Part model, mm, in its own coordinate system. Face numbers are marked on the shaded views. Round coordinates to 2 decimals unless told otherwise and drop trailing zeros. Order: outer loops, then holes, each group sorted by start corner. A loop starts at its lowest first (then second) coordinate and runs counter-clockwise, first axis right, second up. Notation, with made-up numbers: M 69.5,30.5 L 90.5,30.5 A34 ccw 90.5,67.5 Z; hole C 64,63 d2. An arc over 180 degrees is marked long. One line per question, with ' | ' between items.
from build123d import *

# Parameters (mm, degrees)
SKETCH_R  = 11
PAD_DEPTH = 7
FILLET_R  = 2


with BuildPart() as part:
    # Sketch → Pad (new body)
    with BuildSketch(Plane.XY):
        with BuildLine():
            ThreePointArc((-7.384634, -14.193914), (0, -16), (7.384634, -14.193914))
            ThreePointArc((16.615361, -14.193911), (11.999997, -13.065125), (7.384634, -14.193914))
            ThreePointArc((16.615361, -14.193911), (40, 0), (16.615361, 14.193911))
            ThreePointArc((7.384634, 14.193914), (11.999997, 13.065125), (16.615361, 14.193911))
            ThreePointArc((7.384634, 14.193914), (0, 16), (-7.384634, 14.193914))
            ThreePointArc((-16.615359, 14.19391), (-11.999996, 13.065125), (-7.384634, 14.193914))
            ThreePointArc((-16.615359, 14.19391), (-40, 2e-06), (-16.615362, -14.193912))
            ThreePointArc((-7.384634, -14.193914), (-11.999998, -13.065125), (-16.615362, -14.193912))
        make_face()
        with Locations((-24, 0)):
            Circle(SKETCH_R, mode=Mode.SUBTRACT)
        Circle(SKETCH_R, mode=Mode.SUBTRACT)
        with Locations((24, 0)):
            Circle(SKETCH_R, mode=Mode.SUBTRACT)
    extrude(amount=PAD_DEPTH)

    # Fillet
    fillet_edges = [part.edges().sort_by_distance(p)[0] for p in [
        (40, 0, 0),
        (40, 0, 7),
    ]]
    fillet(fillet_edges, radius=FILLET_R)


solid = part.part
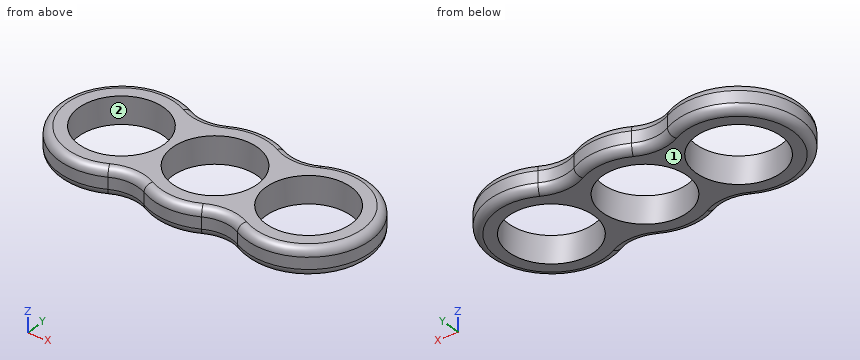
1) Probe line 1 (X direction, y = -3, z = 1.5); line 2 (X direction, y = -4, z = 4); line 3 (Y direction, x = 24, z = 1.75). List the from-to ranges inside material, lowest first. Write a range as [from, to].
The answers:
line 1: x = [-39.65, -34.58], [-13.42, -10.58], [10.58, 13.42], [34.58, 39.65] | line 2: x = [-39.49, -34.25], [-13.75, -10.25], [10.25, 13.75], [34.25, 39.49] | line 3: y = [-15.98, -11], [11, 15.98]
2) Saw through at A-A (x = 0). List the corners of the cut face in (y, z).
The answers:
outline: M -16,2 A2 ccw -14,0 L -11,0 L -11,7 L -14,7 A2 ccw -16,5 Z; M 11,0 L 14,0 A2 ccw 16,2 L 16,5 A2 ccw 14,7 L 11,7 Z
3) Saw through at C-C (y = 9). Give the number of separate pieces and of enclosed holes in the cut face, plus the area to 3 significant figures.
The answers:
separate pieces: 4 | enclosed holes: 0 | area: 251 mm²
4) Two-plate mould, pull along X, no slides. Class the marked faces 1 and 2: released by +X, released by -X, zero draft, split by the parting line, or undercut.
The answers:
face 1: zero draft | face 2: undercut
5) Saw through at B-B (z = 3). List the corners of the cut face in (x, y), plus the area to 3 significant figures.
The answers:
outline: M -16.62,-14.19 A10 cw -7.38,-14.19 A16 ccw 7.38,-14.19 A10 cw 16.62,-14.19 A16 ccw long 16.62,14.19 A10 cw 7.38,14.19 A16 ccw -7.38,14.19 A10 cw -16.62,14.19 A16 ccw long Z; hole C -24,0 d22; hole C 0,0 d22; hole C 24,0 d22 | area: 1,070 mm²
6) Saw through at D-D (z = 6.25). List the corners of the cut face in (x, y), plus the area to 3 significant figures.
The answers:
outline: M -16.82,-13.8 A10.44 cw -7.18,-13.8 A15.56 ccw 7.18,-13.8 A10.44 cw 16.82,-13.8 A15.56 ccw long 16.82,13.8 A10.44 cw 7.18,13.8 A15.56 ccw -7.18,13.8 A10.44 cw -16.82,13.8 A15.56 ccw long Z; hole C -24,0 d22; hole C 0,0 d22; hole C 24,0 d22 | area: 983 mm²
7) Drop a flat-ended pin along its axis: pin 1 (3 mm diameter, centred on x = 20, z = 1.5, fed in from +Y). Give the stop position or say it passes through.
The answers:
pin 1: stops at y = 15.79
